from build123d import *

# Parameters (mm, degrees)
SFAZOWANIE1_SIZE           = 1
SZKIC14_W                  = 16
SZKIC14_H                  = 2
WYTNIJ_WYCI_GNI_CIE1_DEPTH = 3


with BuildPart() as part:
    # Szkic1 → Obrót1 (revolve)
    with BuildSketch(Plane.XY):
        with BuildLine():
            Line((0, 0), (5, 0))
            Line((5, 0), (5, 35.5))
            Line((5, 35.5), (8, 35.5))
            Line((8, 35.5), (8, 37))
            add(Edge.make_bspline(
                [(8, 37), (8, 39.7), (0, 39.7)],
                knots=[0, 0, 0, 1.570796327, 1.570796327, 1.570796327], degree=2, weights=[1, 0.707106781, 1]))
            Line((0, 39.7), (0, 0))
        make_face()
    revolve(axis=Axis((0, 0, 0), (0, 1, 0)))

    # Sfazowanie1
    sfazowanie1_edges = [part.edges().sort_by_distance(p)[0] for p in [
        (-5, 0, 0),
    ]]
    chamfer(sfazowanie1_edges, length=SFAZOWANIE1_SIZE)

    # Szkic14 → Wytnij-wyciągnięcie1 (cut)
    with BuildSketch(Plane(origin=(0, 39.7, 0), x_dir=(1, 0, 0), z_dir=(0, 1, 0))):
        Rectangle(SZKIC14_W, SZKIC14_H)
    extrude(amount=-WYTNIJ_WYCI_GNI_CIE1_DEPTH, mode=Mode.SUBTRACT)


solid = part.part
Input: part model. Units: mm. Frame: model coordinates. A direction names the side the tool comes from. Coordinates: 2 decimals unless noted, no trailing zeros. Loops run counter-clockwise (first coordinate to the right, second up) from the corner with the lowest first, then second, coordinate; pieces in that order, holes last. Notation, with made-up numbers: (69.5, 86) -> (98.5, 86) arc R27 cw to (98.5, 112) -> close; hole circle Ø7 at (-39.5, 28.5). An arc over 180 degrees is marked (long way). Write item = value, one per line. Start each with the question number.
Item 1: Cut plane B-B, the plane y = 7.5. Return loops of the section in (x, z), plus the area to 3 significant figures.
Item 2: First-contact query: P1, Ø0.6, axis at x = -1, z = 0.5, coming from the +Y side; P2, Ø1.5, axis at y = 11.5, z = 4.5, coming from the +X side; P3, Ø1.5, axis at x = 2.5, z = 4, coming from the +Y side; P4, Ø2, axis at y = 18.5, z = -6.5, coming from the -X side. Flat tips, straight axial feed; report the tip coordinate or a pass-through.
Item 3: Reachability of faces 1 (the face through (0.1, 35.5, 5.2)), 2 (the face through (7.39, 36.26, 3.06)), 3 (the face through (0, 38, -1)) from +Z, -Z, +X, -X, +Y, -Y: full face, straight path, thin tool, end or side. Return the list, or none.
Item 4: Material intervals for line 1 (Z direction, x = 0, y = 28); line 2 (X direction, y = 14.5, z = 3); line 3 (Y direction, x = -3.25, z = -0.5), sorted ascending.
Item 5: Mould query, pull axis Z, two halves, no side actions, for faces 4 (the face through (0, 36.7, 0)), 5 (the face through (0, 0, 0)), 6 (the face through (-1.08, 18.49, 4.88)). Classes: pulls with the +Z half, pulls with the -Z half, needs draft (parallel to the pull), parting line crosses it, or undercut.
Item 6: Cut plane A-A, the plane z = 0. Return loops of the section in (x, y).
Ans:
q1.outline = circle Ø10 at (0, 0)
q1.area = 78.5 mm²
q2.P1 = 36.7
q2.P2 = 3.31
q2.P3 = 39.34
q2.P4 = through
q3.face_1 = -Y
q3.face_2 = +Y, -Y
q3.face_3 = +X, -X, +Y
q4.line_1 = -5 to 5
q4.line_2 = -4 to 4
q4.line_3 = 0 to 36.7
q5.face_4 = undercut
q5.face_5 = needs draft
q5.face_6 = parting line crosses it
q6.outline = (-8, 35.5) -> (-5, 35.5) -> (-5, 1) -> (-4, 0) -> (4, 0) -> (5, 1) -> (5, 35.5) -> (8, 35.5) -> (8, 36.7) -> (-8, 36.7) -> close
